Source: CAD feature listing. Evaluate the final solid. Frame: model axes, mm. A direction names the side the tool comes from. Round coordinates to 2 decimals unless told otherwise and drop trailing zeros. Loops run counter-clockwise (first coordinate to the right, second up) from the corner with the lowest first, then second, coordinate; pieces in that order, holes last.
Item 1: First-contact query: P1, Ø1, axis at x = -92.5, z = 17, coming from the +Y side; P2, Ø5, axis at y = 18, z = -16.5, coming from the +X side; P3, Ø6.5, axis at x = -2, y = 34, coming from the -Z side; P4, Ø10, axis at x = -174, z = 5.5, coming from the -Y side. Flat tips, straight axial feed; report the tip coordinate or a pass-through.
Item 2: Section query C-C on x = -53.5. Return loops of the section in (y, z).
Item 3: Ray query, L1, parallel to X at y = 68.5, z = -11.5; L2, parallel to X at y = 67, z = 16; L3, parallel to X at y = 63.5, z = -11.5. Return the intervals inside material, ascending.
Item 4: Pull-direction query (X, two-part tool) for faces 4 (the cylindrical face through (61.692, 65.229, -24.363)), 5 (the flat face through (-11, -12, -21)), 6 (the flat face through (-119, 56, 7.5)); classes: released by +X, released by -X, zero draft, split by the parting line, or undercut.
Item 5: Access query for faces 1 (the flat face through (12, 34, 5)), 2 (the flat face through (-141, 70.3, 2)), 3 (the cylindrical face through (-133.6, 48.8, 17.6)). Directions: +Z, -Z, +X, -X, +Y, -Y. A direction counts if a zero-diameter tool reaches every point of the face in a straight line with its end or side. Return the directions, or none.
Item 6: Section query D-D on x = -116.5. Return loops of the section in (y, z).
Item 7: Section query A-A on y = 0. Return loops of the section in (x, z), then the cut area to 3 significant figures.
Item 8: Section query B-B on x = 0. Return loops of the section in (y, z).
```python
from build123d import *

# Parameters (mm, degrees)
SKETCH_1_R               = 26
EXTRUDE_1_DEPTH          = 21
SKETCH_2_R               = 16
CUT_EXTRUDE_1_DEPTH      = 56.821142948
CUT_EXTRUDE_2_REACH      = 67.695
CUT_EXTRUDE_2_END_RADIUS = 16
SKETCH_3_R               = 5.5
EXTRUDE_2_DEPTH          = 27.5
CUT_EXTRUDE_4_DEPTH      = 212.291599501
CUT_EXTRUDE_4_DEPTH_BACK = 212.291599501
CUT_EXTRUDE_START        = -13.947107552
CUT_EXTRUDE_6_DEPTH      = 13.947107552
SKETCH_7_R               = 5.5
CUT_EXTRUDE_7_DEPTH      = 212.291599501
SKETCH_8_R               = 5.5
CUT_EXTRUDE_8_DEPTH      = 212.291599501
RIB_1_DEPTH              = 10
FILLET_1_R               = 3
RIB_8_REACH              = 202.879
SKETCH_16_WALL_W         = 465.989842276
SKETCH_16_WALL_H         = 10
EXTRUDE_3_DEPTH          = 5
EXTRUDE_4_REACH          = 199.454
EXTRUDE_4_END_RADIUS     = 26


# Read off the part's stored shape, not the designer's step: the extrude step, the rib step
with BuildPart() as part:
    # Sketch 1 → Extrude 1 (new, symmetric)
    with BuildSketch(Plane.XY):
        with Locations(Location((0, 0, 0), (0, 0, 180))):
            Circle(SKETCH_1_R)
    extrude(amount=EXTRUDE_1_DEPTH, both=True)

    # Sketch 2 → Cut-Extrude 1 (cut, through all)
    with BuildSketch(Plane.XY.offset(21)):
        Circle(SKETCH_2_R)
    extrude(amount=-CUT_EXTRUDE_1_DEPTH, mode=Mode.SUBTRACT)

    # Cut-Extrude 2: up to this cylinder (the profile starts outside it)
    cut_extrude_2_end = Plane(origin=(0, 0, 0), z_dir=(0, 0, 1)) * Cylinder(CUT_EXTRUDE_2_END_RADIUS, 168.39, mode=Mode.PRIVATE)
    # Sketch 3 → Cut-Extrude 2 (cut, up to the surface)
    with BuildSketch(Plane(origin=(22.516660498, 13, 0), x_dir=(0, 0, -1), z_dir=(0.8660254037844398, 0.499999999999998, 0)), mode=Mode.PRIVATE) as cut_extrude_2_sk1:
        with Locations(Location((0, 0, 0), (0, 0, 90))):
            Circle(SKETCH_3_R)
    cut_extrude_2_tool1 = extrude(cut_extrude_2_sk1.sketch, amount=-CUT_EXTRUDE_2_REACH, mode=Mode.PRIVATE) - cut_extrude_2_end
    add(cut_extrude_2_tool1.solids().sort_by_distance((22.51666, 13, 0))[0], mode=Mode.SUBTRACT)



with BuildPart() as body_2:
    # Sketch 4 → Extrude 2 (new, symmetric)
    with BuildSketch(Plane.XY):
        with BuildLine():
            Line((-185, 60.3), (-163.497474683, 60.3))
            ThreePointArc((-163.497474683, 60.3), (-161.584057521, 59.919397663), (-159.961940777, 58.835533906))
            Line((-159.961940777, 58.835533906), (-147.213203436, 46.086796564))
            ThreePointArc((-147.213203436, 46.086796564), (-137.480502971, 39.583614025), (-126, 37.3))
            Line((-126, 37.3), (13, 37.3))
            ThreePointArc((13, 37.3), (28, 41.319237886), (38.980762114, 52.3))
            Line((38.980762114, 52.3), (42.475401198, 58.352892448))
            Line((42.475401198, 58.352892448), (65, 58.352892448))
            Line((65, 58.352892448), (65, 72.3))
            Line((65, 72.3), (38.980762114, 72.3))
            Line((38.980762114, 72.3), (30.320508076, 57.3))
            ThreePointArc((30.320508076, 57.3), (23, 49.979491924), (13, 47.3))
            Line((13, 47.3), (-126, 47.3))
            ThreePointArc((-126, 47.3), (-133.653668647, 48.82240935), (-140.142135624, 53.157864376))
            Line((-140.142135624, 53.157864376), (-159.284271247, 72.3))
            Line((-159.284271247, 72.3), (-185, 72.3))
            Line((-185, 72.3), (-185, 60.3))
        make_face()
    extrude(amount=EXTRUDE_2_DEPTH, both=True)

    # Sketch 5 → Cut-Extrude 4 (cut, two sides: drawn at the far end of the back side and taken through both)
    with BuildSketch(Plane(origin=(0, 72.3, 0), x_dir=(1, 0, 0), z_dir=(0, 1, 0)).offset(-CUT_EXTRUDE_4_DEPTH_BACK)):
        with BuildLine():
            Line((-7.168790364, 499.369918589), (-174, 27.5))
            Line((-174, 27.5), (-184.370899457, -1.833333333))
            ThreePointArc((-184.370899457, -1.833333333), (-184.953601074, -6.509268805), (-183.526279442, -11))
            Line((-183.526279442, -11), (-174, -27.5))
            Line((-174, -27.5), (76.246814454, -460.940197067))
            Line((76.246814454, -460.940197067), (-920.985347946, -547.562968831))
            Line((-920.985347946, -547.562968831), (-1004.400952764, 412.747146826))
            Line((-1004.400952764, 412.747146826), (-7.168790364, 499.369918589))
        make_face()
    extrude(amount=CUT_EXTRUDE_4_DEPTH + CUT_EXTRUDE_4_DEPTH_BACK, mode=Mode.SUBTRACT)

    # Cut-Extrude 6 outline → Cut-Extrude 6 (cut)
    with BuildSketch(Plane(origin=(0, 72.3, 0), x_dir=(1, 0, 0), z_dir=(0, 1, 0)).offset(CUT_EXTRUDE_START)):
        with BuildLine():
            Line((65, -27.5), (65, -16.5))
            ThreePointArc((65, -16.5), (61.778174593, -24.278174593), (54, -27.5))
            Line((54, -27.5), (65, -27.5))
        make_face()
        with BuildLine():
            ThreePointArc((54, 27.5), (61.778174593, 24.278174593), (65, 16.5))
            Line((65, 16.5), (65, 27.5))
            Line((65, 27.5), (54, 27.5))
        make_face()
    extrude(amount=CUT_EXTRUDE_6_DEPTH, mode=Mode.SUBTRACT)

    # Sketch 7 → Cut-Extrude 7 (cut, through all)
    with BuildSketch(Plane(origin=(0, 72.3, 0), x_dir=(1, 0, 0), z_dir=(0, 1, 0))):
        with Locations(Location((54, 16.5, 0), (0, 0, 270))):
            Circle(SKETCH_7_R)
    cut_extrude_7 = extrude(amount=-CUT_EXTRUDE_7_DEPTH, mode=Mode.SUBTRACT)

    # Mirror 1: Cut-Extrude 7 across plane
    add(cut_extrude_7.mirror(Plane.XY), mode=Mode.SUBTRACT)

    # Sketch 8 → Cut-Extrude 8 (cut, through all)
    with BuildSketch(Plane(origin=(0, 72.3, 0), x_dir=(1, 0, 0), z_dir=(0, 1, 0))):
        with Locations(Location((-174, -5.5, 0), (0, 0, 270))):
            Circle(SKETCH_8_R)
    extrude(amount=-CUT_EXTRUDE_8_DEPTH, mode=Mode.SUBTRACT)

    # Sketch 10 → 8.0mm _1 (revolve, cut)
    with BuildSketch(Plane(origin=(54, 72.3, -1.5), x_dir=(0, 0, 1), z_dir=(1, 0, 0))):
        Polygon((0, 0), (0, 13.948107552), (4, 13.948107552), (4, 1), (5, 0), align=None)
    revolve(axis=Axis((54, 78.65, -1.5), (0, -1, 0)), mode=Mode.SUBTRACT)

    # Sketch 12 → 8.0mm _2 (revolve, cut)
    with BuildSketch(Plane(origin=(-169, 72.3, -11.5), x_dir=(0, 0, 1), z_dir=(1, 0, 0))):
        Polygon((0, 0), (0, 12.001), (4, 12.001), (4, 1), (5, 0), align=None)
    revolve(axis=Axis((-169, 78.65, -11.5), (0, -1, 0)), mode=Mode.SUBTRACT)

    # Rib 1 outline → Rib 1 (add)
    with BuildSketch(Plane.XY.offset(-2.5)):
        with BuildLine():
            Line((-56, 47.3), (-126, 70.3))
            Line((-126, 70.3), (-157.284271247, 70.3))
            Line((-157.284271247, 70.3), (-140.142135624, 53.157864376))
            ThreePointArc((-140.142135624, 53.157864376), (-133.653668647, 48.82240935), (-126, 47.3))
            Line((-126, 47.3), (-56, 47.3))
        make_face()
    extrude(amount=RIB_1_DEPTH)

    # Fillet 1
    fillet_1_edges = [body_2.edges().sort_by_distance(p)[0] for p in [
        (-174, 66.3, -27.5),
        (-174, 66.3, 27.5),
    ]]
    fillet(fillet_1_edges, radius=FILLET_1_R)

    # Sketch 16 wall → Rib 8 (add, up to next)
    with BuildSketch(Plane(origin=(8.913030787, 58.8, -2.5), x_dir=(0.929197613161, 0.369583273019, 0), z_dir=(-0.369583273019, 0.929197613161, 0)), mode=Mode.PRIVATE) as rib_8_sk1:
        with Locations((0, -5)):
            Rectangle(SKETCH_16_WALL_W, SKETCH_16_WALL_H)
    rib_8_tool1 = extrude(rib_8_sk1.sketch, amount=-RIB_8_REACH, mode=Mode.PRIVATE) - body_2.part
    add(rib_8_tool1.solids().sort_by_distance((8.913030787, 58.8, -2.5))[0])


with BuildPart() as part_1:
    add(part.part)

    add(body_2.part)  # Extrude 3 merges body 2
    # Sketch 17 → Extrude 3 (add, symmetric)
    with BuildSketch(Plane.XY):
        with BuildLine():
            Line((-11.614576615, -23.261590875), (-137.480502971, 39.583614025))
            ThreePointArc((-137.480502971, 39.583614025), (-131.85270966, 37.876441588), (-126, 37.3))
            Line((-126, 37.3), (13, 37.3))
            ThreePointArc((13, 37.3), (21.130139995, 38.422658993), (28.651788339, 41.706611756))
            Line((28.651788339, 41.706611756), (10, 30.3))
            ThreePointArc((10, 30.3), (8.254139309, 26.922225109), (10.440740808, 23.811571375))
            ThreePointArc((10.440740808, 23.811571375), (-23.543897802, 11.031086814), (-11.614576615, -23.261590875))
        make_face()
    extrude(amount=EXTRUDE_3_DEPTH, both=True)

    # Extrude 4: up to this cylinder (the profile starts outside it)
    extrude_4_end = Plane(origin=(0, 0, 0), z_dir=(0, 0, -1)) * Cylinder(EXTRUDE_4_END_RADIUS, 451.908, mode=Mode.PRIVATE)
    # Sketch 19 → Extrude 4 (add, up to the surface)
    with BuildSketch(Plane.XZ.offset(-37.3), mode=Mode.PRIVATE) as extrude_4_sk1:
        Polygon((-4, -19), (4, -19), (7.350212633, 0), (4, 19), (-4, 19), (-7.350212633, 0), align=None)
    extrude_4_tool1 = extrude(extrude_4_sk1.sketch, amount=EXTRUDE_4_REACH, mode=Mode.PRIVATE) - extrude_4_end
    add(extrude_4_tool1.solids().sort_by_distance((0, 37.3, 0))[0])


solid = part_1.part
```
Data:
1. P1: stops at y = 47.3
1. P2: stops at x = 20.87
1. P3: stops at z = -19
1. P4: passes through
2. outline: (-2.35, -5) - (37.3, -5) - (37.3, -27.5) - (47.3, -27.5) - (47.3, 27.5) - (37.3, 27.5) - (37.3, 5) - (-2.35, 5) - close
3. L1: x = -179.66 to -173, -165 to -155.48, 36.79 to 51.71, 56.29 to 65
3. L2: x = -180.64 to -153.98, 35.92 to 48.52, 59.48 to 65
3. L3: x = -179.66 to -173, -165 to -150.48, 33.9 to 51.71, 56.29 to 65
4. face 4: released by +X
4. face 5: zero draft
4. face 6: undercut
5. face 1: +Z, +X
5. face 2: +Z, -Z, +Y
5. face 3: +Z, +Y
6. outline: (29.11, -5) - (37.3, -5) - (37.3, -27.5) - (47.3, -27.5) - (47.3, -2.5) - (67.18, -2.5) - (67.18, 7.5) - (47.3, 7.5) - (47.3, 27.5) - (37.3, 27.5) - (37.3, 5) - (29.11, 5) - close
7. outline: (-58.2, -5) - (-26, -5) - (-26, -21) - (-16, -21) - (-16, 21) - (-26, 21) - (-26, 5) - (-58.2, 5) - close; (16, -21) - (26, -21) - (26, 21) - (16, 21) - close
7. area: 1,160 mm2
8. outline: (-26, -21) - (-16, -21) - (-16, 21) - (-26, 21) - close; (16, -21) - (26, -21) - (26, -19) - (37.3, -19) - (37.3, -27.5) - (47.3, -27.5) - (47.3, -2.5) - (55.25, -2.5) - (55.25, 7.5) - (47.3, 7.5) - (47.3, 27.5) - (37.3, 27.5) - (37.3, 19) - (26, 19) - (26, 21) - (16, 21) - close
